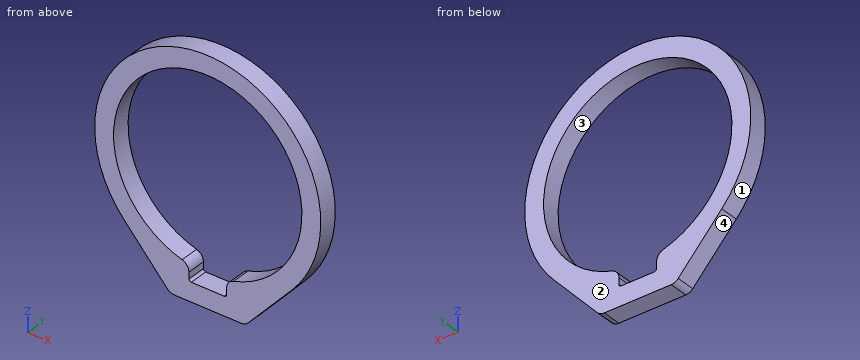
from build123d import *

# Parameters (mm, degrees)
BOSS_EXTRUDE1_DEPTH = 6.35
FILLET1_R           = 0.79375
FILLET3_R           = 3.175


with BuildPart() as part:
    # Sketch1 → Boss-Extrude1 (new body)
    with BuildSketch(Plane(origin=(0, 0, 0), x_dir=(1, 0, 0), z_dir=(0, 1, 0))):
        with BuildLine():
            Line((-12.7, 42.8625), (-28.334044467, 25.471394232))
            ThreePointArc((-28.334044467, 25.471394232), (0, -38.1), (28.334044467, 25.471394232))
            Line((28.334044467, 25.471394232), (12.7, 42.8625))
            Line((12.7, 42.8625), (-12.7, 42.8625))
        make_face()
        with BuildLine():
            Line((-6.35, 36.5125), (6.35, 36.5125))
            Line((6.35, 36.5125), (6.35, 31.108519733))
            ThreePointArc((6.35, 31.108519733), (0, -31.75), (-6.35, 31.108519733))
            Line((-6.35, 31.108519733), (-6.35, 36.5125))
        make_face(mode=Mode.SUBTRACT)
    extrude(amount=BOSS_EXTRUDE1_DEPTH)

    # Fillet1
    fillet1_edges = [part.edges().sort_by_distance(p)[0] for p in [
        (-6.35, 3.175, -36.5125),
        (6.35, 3.175, -36.5125),
    ]]
    fillet(fillet1_edges, radius=FILLET1_R)

    # Fillet3
    fillet3_edges = [part.edges().sort_by_distance(p)[0] for p in [
        (-6.35, 3.175, -31.108519733),
        (6.35, 3.175, -31.108519733),
        (-12.7, 3.175, -42.8625),
        (12.7, 3.175, -42.8625),
    ]]
    fillet(fillet3_edges, radius=FILLET3_R)


solid = part.part
Could you check a few things on this model? Use its own coordinates, in mm. Face numbers are marked on the shaded views. Coordinates: 2 decimals unless noted, no trailing zeros. Order: outer loops, then holes, each group sorted by start corner. A loop starts at its lowest first (then second) coordinate and runs counter-clockwise, first axis right, second up.
Q1. Please list where these lines run through material, in increasing order: L1, parallel to Z at x = -1, y = 4.25; L2, parallel to X at y = 1.5, z = 0; L3, parallel to Z at x = 20.5, y = 2.
Q2. Thinking about a two-plate mould opening in X: for the marked faces 1, 2, 3 and 4, which applies, released by +X, released by -X, zero draft, split by the parting line, or undercut?
Q3. Will these pins go through, and if not, where does the flat tip stop? pin 1 (1 mm diameter, centred on y = 3.5, z = 29.5, fed in from +X); pin 2 (2.5 mm diameter, centred on y = 4, z = -34.5, fed in from -X); pin 3 (1.1 mm diameter, centred on y = 3, z = -35, fed in from +X).
Q4. Suppose I cut it at B-B on z = 0. Please give me the cut outline in (x, y), and give its area (3 significant figures).
Q5. Suppose I cut it at A-A on x = 0. Please give me the cut outline in (y, z), and give its area (3 significant figures).
Answer:
1. L1: z = -42.86 to -36.51, 31.73 to 38.09
1. L2: x = -38.1 to -31.75, 31.75 to 38.1
1. L3: z = -34.19 to -24.24, 24.24 to 32.11
2. face 1: split by the parting line
2. face 2: zero draft
2. face 3: undercut
2. face 4: released by -X
3. pin 1: stops at x = 24.71
3. pin 2: stops at x = -21.34
3. pin 3: stops at x = 20.26
4. outline: (-38.1, 0) - (-31.75, 0) - (-31.75, 6.35) - (-38.1, 6.35) - close; (31.75, 0) - (38.1, 0) - (38.1, 6.35) - (31.75, 6.35) - close
4. area: 80.6 mm2
5. outline: (0, -42.86) - (6.35, -42.86) - (6.35, -36.51) - (0, -36.51) - close; (0, 31.75) - (6.35, 31.75) - (6.35, 38.1) - (0, 38.1) - close
5. area: 80.6 mm2
